Verification items for the finished model (mm, model axes). A direction names the side the tool comes from. Coordinates: 2 decimals unless noted, no trailing zeros. Order: outer loops, then holes, each group sorted by start corner. A loop starts at its lowest first (then second) coordinate and runs counter-clockwise, first axis right, second up.
Q1. Thickness scan on line 1 (X direction, y = -40.5, z = 60); line 2 (Z direction, x = 70, y = -37.25); line 3 (Z direction, x = 77.25, y = -36.25). Record the ranges inside material, lowest first.
Q2. Cross-section at B-B, the plane z = 109. Record the boundary of the cut face in (x, y).
Q3. Cross-section at A-A, the plane x = 71.2. Record the boundary of the cut face in (y, z), and give its area (3 significant figures).
Q4. Set-up check for faces 5 (the flat face through (76.4, -38, 112)), 6 (the cylindrical face through (71.1, -41.2, 4.2)), 7 (the cylindrical face through (61.3, -37.6, 25.1)), 8 (the cylindrical face through (71.1, -37.6, 4.2)), 9 (the cylindrical face through (71.1, -34, 245.8)): record each of +Z, -Z, +X, -X, +Y, -Y from which the full face is reachable in a straight line by a thin tool's end or side.
Q5. Draft check along Z on faces 1 (the flat face through (71, -33.3, 4)), 2 (the cylindrical face through (62.9, -37.6, 25.1)), 3 (the cylindrical face through (71.3, -34, 4.2)), 4 (the cylindrical face through (71.3, -37.6, 245.8)). Enter one of: pulls with the +Z half, pulls with the -Z half, needs draft (parallel to the pull), parting line crosses it, or undercut.
Q6. Depth check by flat-ended pin: P1, Ø3, axis at x = 75.5, y = -38.5, coming from the -Z side; P2, Ø0.6, axis at y = -34, z = 236.5, coming from the -X side; P3, Ø1.4, axis at y = -41, z = 237.5, coming from the -X side; P4, Ø7.5, axis at x = 75, z = 9.5, coming from the +Y side. Enter the tip coordinate at first touch or a pass-through.
Q7. Cross-section at C-C, the plane y = -37.5. Record the boundary of the cut face in (x, z), and give its area (3 significant figures).
from build123d import *

# Parameters (mm, degrees)
PAD004_DEPTH      = 3
PAD006_DEPTH      = 1.3
PAD006_DEPTH_BACK = 0.01
PAD007_DEPTH      = 1.3
PAD007_DEPTH_BACK = 0.001


with BuildPart() as part:
    # Sketch018 → Pad004 (new body, symmetric)
    with BuildSketch(Plane(origin=(71.2, -37.6, 0), x_dir=(1, 0, 0), z_dir=(0, -1, 0))):
        with BuildLine():
            ThreePointArc((-6.8, 11), (0, 4.2), (6.8, 11))
            Line((6.8, 11), (6.8, 216.735014))
            ThreePointArc((8.23, 220.316508), (7.170714, 218.663225), (6.8, 216.735014))
            ThreePointArc((8.23, 220.316508), (10.1, 225), (8.23, 229.683492))
            ThreePointArc((6.8, 233.264986), (7.170714, 231.336775), (8.23, 229.683492))
            Line((6.8, 239), (6.8, 233.264986))
            ThreePointArc((6.8, 239), (0, 245.8), (-6.8, 239))
            Line((-6.8, 33.049224), (-6.8, 239))
            ThreePointArc((-8.143333, 29.561227), (-7.147441, 31.180356), (-6.8, 33.049224))
            ThreePointArc((-8.143333, 29.561227), (-9.9, 25), (-8.143333, 20.438773))
            ThreePointArc((-6.8, 16.950776), (-7.147441, 18.819644), (-8.143333, 20.438773))
            Line((-6.8, 11), (-6.8, 16.950776))
        make_face()
        with BuildLine():
            ThreePointArc((-5.2, 11), (0, 5.8), (5.2, 11))
            Line((5.2, 11), (5.2, 216.735014))
            ThreePointArc((7.07, 221.418506), (5.68478, 219.256521), (5.2, 216.735014))
            ThreePointArc((7.07, 221.418506), (8.5, 225), (7.07, 228.581494))
            ThreePointArc((5.2, 233.264986), (5.68478, 230.743479), (7.07, 228.581494))
            Line((5.2, 239), (5.2, 233.264986))
            ThreePointArc((5.2, 239), (0, 244.2), (-5.2, 239))
            Line((-5.2, 33.049224), (-5.2, 239))
            ThreePointArc((-6.956667, 28.487997), (-5.654345, 30.60532), (-5.2, 33.049224))
            ThreePointArc((-6.956667, 28.487997), (-8.3, 25), (-6.956667, 21.512003))
            ThreePointArc((-5.2, 16.950776), (-5.654345, 19.39468), (-6.956667, 21.512003))
            Line((-5.2, 11), (-5.2, 16.950776))
        make_face(mode=Mode.SUBTRACT)
    extrude(amount=PAD004_DEPTH, both=True)

    # Sketch020 (on Face26 of Pad004) → Pad006 (join, two sides)
    with BuildSketch(Plane.XZ.offset(40.6)) as pad006_sk:
        with BuildLine():
            ThreePointArc((64.4, 11), (71.2, 4.2), (78, 11))
            Line((78, 17.196773), (78, 11))
            ThreePointArc((64.4, 17.196773), (71.2, 1.8), (78, 17.196773))
            Line((64.4, 17.196773), (64.4, 11))
        make_face()
        with BuildLine():
            ThreePointArc((78, 239), (71.2, 245.8), (64.4, 239))
            Line((64.4, 232.803227), (64.4, 239))
            ThreePointArc((78, 232.803227), (71.2, 248.2), (64.4, 232.803227))
            Line((78, 232.803227), (78, 239))
        make_face()
    extrude(amount=PAD006_DEPTH)
    extrude(pad006_sk.sketch, amount=-PAD006_DEPTH_BACK)

    # Sketch021 (on Face2 of Pad006) → Pad007 (join, two sides)
    with BuildSketch(Plane(origin=(0, -34.6, 0), x_dir=(1, 0, 0), z_dir=(0, 1, 0))) as pad007_sk:
        with BuildLine():
            ThreePointArc((78, -11), (71.2, -4.2), (64.4, -11))
            Line((64.4, -17.196773), (64.4, -11))
            ThreePointArc((78, -17.196773), (71.2, -1.8), (64.4, -17.196773))
            Line((78, -17.196773), (78, -11))
        make_face()
        with BuildLine():
            ThreePointArc((64.4, -239), (71.2, -245.8), (78, -239))
            Line((78, -232.803227), (78, -239))
            ThreePointArc((64.4, -232.803227), (71.2, -248.2), (78, -232.803227))
            Line((64.4, -232.803227), (64.4, -239))
        make_face()
    extrude(amount=PAD007_DEPTH)
    extrude(pad007_sk.sketch, amount=-PAD007_DEPTH_BACK)


solid = part.part
Check values:
1. line 1: x = 64.4 to 66, 76.4 to 78
1. line 2: z = 4.31 to 5.94, 244.06 to 245.69
1. line 3: z = 7.9 to 220.03, 229.97 to 242.1
2. outline: (64.4, -40.6) - (66, -40.6) - (66, -34.6) - (64.4, -34.6) - close; (76.4, -40.6) - (78, -40.6) - (78, -34.6) - (76.4, -34.6) - close
3. outline: (-41.9, 1.8) - (-40.59, 1.8) - (-40.59, 4.2) - (-34.6, 4.2) - (-34.6, 1.8) - (-33.3, 1.8) - (-33.3, 4.2) - (-34.6, 4.2) - (-34.6, 5.8) - (-40.6, 5.8) - (-40.6, 4.2) - (-41.9, 4.2) - close; (-41.9, 245.8) - (-40.6, 245.8) - (-40.6, 244.2) - (-34.6, 244.2) - (-34.6, 245.8) - (-33.3, 245.8) - (-33.3, 248.2) - (-34.6, 248.2) - (-34.6, 245.8) - (-40.59, 245.8) - (-40.59, 248.2) - (-41.9, 248.2) - close
3. area: 31.7 mm2
4. face 5: +Y, -Y
4. face 6: -Y
4. face 7: -X, +Y, -Y
4. face 8: -Z
4. face 9: +Y
5. face 1: needs draft
5. face 2: undercut
5. face 3: undercut
5. face 4: pulls with the +Z half
6. P1: stops at z = 4.8
6. P2: stops at x = 62.27
6. P3: stops at x = 62.03
6. P4: stops at y = -33.3
7. outline: (63.06, 20.44) arc R5.2 cw to (64.4, 16.95) - (64.4, 11) arc R6.8 ccw to (78, 11) - (78, 216.74) arc R5.2 cw to (79.43, 220.32) arc R6.8 ccw to (79.43, 229.68) arc R5.2 cw to (78, 233.26) - (78, 239) arc R6.8 ccw to (64.4, 239) - (64.4, 33.05) arc R5.2 cw to (63.06, 29.56) arc R6.8 ccw to start; hole (64.24, 21.51) arc R6.8 cw to (66, 16.95) - (66, 11) arc R5.2 ccw to (76.4, 11) - (76.4, 216.74) arc R6.8 cw to (78.27, 221.42) arc R5.2 ccw to (78.27, 228.58) arc R6.8 cw to (76.4, 233.26) - (76.4, 239) arc R5.2 ccw to (66, 239) - (66, 33.05) arc R6.8 cw to (64.24, 28.49) arc R5.2 ccw to start
7. area: 795 mm2
